Autodesk Inventor part; units mm, degrees
ref_plane "YZ Plane" through (0, 0, 0) normal (1, 0, 0) x (0, 1, 0)
ref_plane "XZ Plane" through (0, 0, 0) normal (0, 1, 0) x (-1, 0, 0)
ref_plane "XY Plane" through (0, 0, 0) normal (0, 0, 1) x (1, 0, 0)
sketch "Sketch1" plane through (0, 0, 0) normal (0, 1, 0) x (-1, 0, 0)
  circle A0 centre (0, 0) radius 120
  circle A1 centre (-9, 10) radius 1
  circle A2 centre (-9, -10) radius 1
  circle A3 centre (-29, -10) radius 1
  circle A4 centre (-29, 10) radius 1
  arc A5 (-8.0467, -7.5) -> (-8.0467, 7.5) centre (0, 0) ccw
  line L0 (-9, -7.5) -> (-8.0467, -7.5)
  line L1 (-9, -7.5) -> (-11, -7.5)
  line L2 (-11, -7.5) -> (-11, -11.5)
  line L3 (-29, -10) -> (-26, -10)
  line L4 (-11, -11.5) -> (-26, -11.5)
  line L5 (-26, -11.5) -> (-26, -7.5)
  line L6 (-26, -7.5) -> (-35, -7.5)
  line L7 (-35, -7.5) -> (-35, 0)
  line L8 (-9, 7.5) -> (-8.0467, 7.5)
  line L9 (-9, 7.5) -> (-11, 7.5)
  line L10 (-11, 7.5) -> (-11, 11.5)
  line L11 (-11, 11.5) -> (-26, 11.5)
  line L12 (-26, 11.5) -> (-26, 7.5)
  line L13 (-26, 7.5) -> (-35, 7.5)
  line L14 (-35, 7.5) -> (-35, 0)
  dimension "d0" = 240
  dimension "d5" = 2
  dimension "d6" = 2
  dimension "d7" = 2
  dimension "d8" = 2
  dimension "d9" = 22
  dimension "d12" = 2
  dimension "d13" = 3
  dimension "d14" = 4
  dimension "d15" = 9
extrude "Extrusion1" add sketch "Sketch1" along normal blind 2
sketch "Sketch4" plane through (0, 2, 0) normal (0, 1, 0) x (1, 0, 0)
  circle A0 centre (0, 0) radius 60
  circle A1 centre (0, 0) radius 120.1645
  dimension "d28" = 120
  dimension "d29" = 240.329
extrude "Extrusion3" cut sketch "Sketch4" against normal blind 12
sketch "Sketch5" plane through (0, 2, 0) normal (0, 1, 0) x (1, 0, 0)
  circle A0 centre (0, 0) radius 28
  line L0 (0, 0) -> (19.799, 19.799)
  line L1 (0, 0) -> (28, 0) construction
  line L2 (19.799, 19.799) -> (-19.799, 19.799)
  line L3 (-19.799, 19.799) -> (-19.799, -19.799)
  line L4 (-19.799, -19.799) -> (19.799, -19.799)
  circle A1 centre (-19.799, -19.799) radius 3
  circle A2 centre (-19.799, 19.799) radius 3
  circle A3 centre (19.799, 19.799) radius 3
  circle A4 centre (19.799, -19.799) radius 3
  line L5 (19.799, 19.799) -> (42.4264, 42.4264)
  circle A5 centre (0, 0) radius 80
  circle A6 centre (0, 0) radius 60
  dimension "d56" = 56
  dimension "d57" = 45
  dimension "d58" = 6
  dimension "d59" = 6
  dimension "d60" = 6
  dimension "d62" = 6
  dimension "d63" = 32
  dimension "d64" = 160
extrude "Extrusion4" add sketch "Sketch5" against normal blind 2 contours A5
sketch "Sketch8" plane through (0, 2, 0) normal (0, 1, 0) x (1, 0, 0)
  circle A0 centre (-42.4264, -42.4264) radius 3
  arc A1 (-53.7401, -31.1127) -> (-31.1127, -53.7401) centre (-42.4264, -42.4264) ccw
  circle A2 centre (42.4264, -42.4264) radius 3
  arc A3 (31.1127, -53.7401) -> (53.7401, -31.1127) centre (42.4264, -42.4264) ccw
  circle A4 centre (42.4264, 42.4264) radius 3
  arc A5 (53.7401, 31.1127) -> (31.1127, 53.7401) centre (42.4264, 42.4264) ccw
  circle A6 centre (-42.4264, 42.4264) radius 3
  arc A7 (-31.1127, 53.7401) -> (-53.7401, 31.1127) centre (-42.4264, 42.4264) ccw
  line L0 (-53.7401, 31.1127) -> (-33.9411, 11.3137)
  line L1 (11.3137, -33.9411) -> (31.1127, -53.7401)
  line L2 (-53.7401, -31.1127) -> (-33.9411, -11.3137)
  line L3 (11.3137, 33.9411) -> (31.1127, 53.7401)
  line L4 (-31.1127, 53.7401) -> (-11.3137, 33.9411)
  line L5 (33.9411, -11.3137) -> (53.7401, -31.1127)
  line L6 (-31.1127, -53.7401) -> (-11.3137, -33.9411)
  line L7 (33.9411, 11.3137) -> (53.7401, 31.1127)
  arc A8 (11.3137, -33.9411) -> (-11.3137, -33.9411) centre (0, -45.2548) ccw
  arc A9 (33.9411, 11.3137) -> (33.9411, -11.3137) centre (45.2548, 0) ccw
  arc A10 (-11.3137, 33.9411) -> (11.3137, 33.9411) centre (0, 45.2548) ccw
  arc A11 (-33.9411, -11.3137) -> (-33.9411, 11.3137) centre (-45.2548, 0) ccw
  circle A12 centre (0, 0) radius 80
extrude "Extrusion7" cut sketch "Sketch8" against normal blind 2 contours A12
sketch "Sketch10" plane through (0, 2, 0) normal (0, 1, 0) x (1, 0, 0)
  line L0 (0, 0) -> (60, 0) construction
  circle A0 centre (42.4264, -42.4264) radius 1.5
  circle A1 centre (19.799, -19.799) radius 1.5
  circle A2 centre (19.799, 19.799) radius 1.5
  circle A3 centre (42.4264, 42.4264) radius 1.5
  circle A4 centre (-19.799, 19.799) radius 1.5
  circle A5 centre (-42.4264, 42.4264) radius 1.5
  circle A6 centre (-19.799, -19.799) radius 1.5
  circle A7 centre (-42.4264, -42.4264) radius 1.5
  dimension "d128" = 3
  dimension "d129" = 3
  dimension "d132" = 360
extrude "Extrusion9" cut sketch "Sketch10" against normal blind 10
properties part number "platform 1"
For this review, take the finished solid that the model builds, in its own axes (mm). A direction names the side the tool comes from. Round coordinates to 2 decimals unless told otherwise and drop trailing zeros. Write each loop counter-clockwise with the first axis right and the second up, starting at its lowest first coordinate (ties: lowest second). Pieces come first, ordered by that corner, then holes. Notation, with made-up numbers: (66, 70) -> (101, 70) arc R31 ccw to (101, 97) -> close; hole circle Ø5 at (21, -17.5). An arc over 180 degrees is marked (long way). Put each result on its own line as item: value.
Q1. The part is to be moulded in two halves that separate along Z. For faces 1 (the cylindrical face through (32.41, 1.01, -9.54)), 2 (the flat face through (-14, 0, -1)), 3 (the flat face through (-21.35, 1.01, -43.98)), say which applies: released by +Z, released by -Z, zero draft, split by the parting line, or undercut.
Determined:
face 1: undercut
face 2: zero draft
face 3: released by -Z
Q2. Consider section B-B on z = -35.5. State the section outline as (x, y) points, and give its area (3 significant figures).
Determined:
outline: (-56.85, 0) -> (-12.87, 0) -> (-12.87, 2) -> (-56.85, 2) -> close; (12.87, 0) -> (56.85, 0) -> (56.85, 2) -> (12.87, 2) -> close
area: 176 mm^2
Q3. Consider section A-A on x = 0. State the section outline as (y, z) points, and give its area (3 significant figures).
Determined:
outline: (0, -29.25) -> (2, -29.25) -> (2, -11) -> (0, -11) -> close; (0, 11) -> (2, 11) -> (2, 29.25) -> (0, 29.25) -> close
area: 73.0 mm^2
Q4. Consider section C-C on z = 0. State the section outline as (x, y) points.
Determined:
outline: (-29.25, 0) -> (-11, 0) -> (-11, 2) -> (-29.25, 2) -> close
Q5. To check wall thickness, follow L1, parallel to X at y = 1.5, z = -8.5; L2, parallel to X at y = 0.95, z = -20; L3, parallel to Z at x = 29, y = 0.8. State the ranges of each line that lie inside material, in increasing order. Write a range as [from, to].
Determined:
L1: x = [-31.7, -6.98], [6.98, 11], [26, 31.7]
L2: x = [-42.63, -21.29], [-18.31, 18.31], [21.29, 42.63]
L3: z = [-51.63, -11], [-9, -7.5], [7.5, 9], [11, 51.63]
Q6. Machinability: for faces 4 (the flat face through (-43.98, 1.01, 21.35)), 5 (the flat face through (21.07, 1.01, 43.7)), 6 (the flat face through (-14, 2, -1)), 7 (the flat face through (21.07, 1.01, -43.7)), 8 (the cylindrical face through (32.369, 1.014, 9.485)), which of the approach directions +Z, -Z, +X, -X, +Y, -Y give a long, thin tool a straight path to every point of the face, cutting with its end or side? Answer none if there is none.
Determined:
face 4: -X, +Y, -Y
face 5: +Z, +Y, -Y
face 6: +Z, -Z, +X, -X, +Y
face 7: -Z, +Y, -Y
face 8: +X, +Y, -Y
Q7. Consider section D-D on y = 0.4. Give the number of separate pieces and of enclosed holes in the cut face, and give its area (3 significant figures).
Determined:
separate pieces: 1
enclosed holes: 12
area: 7,620 mm^2
Q8. Clearance check with flat-ended pins moving along their axes: pin 1 Ø1 at (x, y) = (16, 1) entering from -Z; pin 2 Ø4 at (x, z) = (-42.43, 42.43) entering from -Y; pin 3 Ø0.6 at (x, y) = (29, 1) entering from +Z; pin 4 Ø1 at (y, z) = (1, -45) entering from -X. State where each tip first meets the part, or that it passes through.
Determined:
pin 1: stops at z = -39.13
pin 2: stops at y = 0
pin 3: stops at z = 51.93
pin 4: stops at x = -58.29
